from build123d import *

# Parameters (mm, degrees)
BOSS_EXTRU_1_DEPTH = 100
ESQUISSE2_W        = 20
ESQUISSE2_H        = 60
BOSS_EXTRU_2_DEPTH = 40
CONG_1_R           = 10
CONG_2_R           = 10
CONG_3_R           = 10


with BuildPart() as part:
    # Esquisse1 → Boss.-Extru.1 (new body)
    with BuildSketch(Plane.XY):
        with BuildLine():
            Line((90, -10), (90, 10))
            Line((90, 10), (31.994888516, 10))
            ThreePointArc((31.994888516, 10), (10.78168508, 18.786796564), (1.994888516, 40))
            Line((1.994888516, 40), (1.994888516, 88.375065612))
            Line((1.994888516, 88.375065612), (-83.555876775, 88.375065612))
            ThreePointArc((-83.555876775, 88.375065612), (-90.626944587, 85.446133424), (-93.555876775, 78.375065612))
            Line((-93.555876775, 78.375065612), (-93.555876775, 30))
            Line((-93.555876775, 30), (-22.555876775, 30))
            Line((-22.555876775, 30), (-22.555876775, -30))
            Line((-22.555876775, -30), (-93.555876775, -30))
            Line((-93.555876775, -30), (-93.555876775, -78.375065612))
            ThreePointArc((-93.555876775, -78.375065612), (-90.626944587, -85.446133424), (-83.555876775, -88.375065612))
            Line((-83.555876775, -88.375065612), (1.994888516, -88.375065612))
            Line((1.994888516, -88.375065612), (1.994888516, -40))
            ThreePointArc((1.994888516, -40), (10.78168508, -18.786796564), (31.994888516, -10))
            Line((31.994888516, -10), (90, -10))
        make_face()
    extrude(amount=BOSS_EXTRU_1_DEPTH)

    # Esquisse2 → Boss.-Extru.2 (add)
    with BuildSketch(Plane.ZY.offset(22.555876775)):
        with Locations((90, 0)):
            Rectangle(ESQUISSE2_W, ESQUISSE2_H)
    extrude(amount=BOSS_EXTRU_2_DEPTH)

    # Congé1
    cong_1_edges = [part.edges().sort_by_distance(p)[0] for p in [
        (1.994888516, -88.375065612, 50),
    ]]
    fillet(cong_1_edges, radius=CONG_1_R)

    # Congé2
    cong_2_edges = [part.edges().sort_by_distance(p)[0] for p in [
        (1.994888516, 88.375065612, 50),
    ]]
    fillet(cong_2_edges, radius=CONG_2_R)

    # Congé3
    cong_3_edges = [part.edges().sort_by_distance(p)[0] for p in [
        (90, -10, 50),
        (90, 10, 50),
    ]]
    fillet(cong_3_edges, radius=CONG_3_R - 0.0001)  # a hair under: the kernel refuses the full size


solid = part.part
The listing builds one solid part. Answer for the finished solid, in the listing's coordinates (mm). A direction names the side the tool comes from. Give positions to 0.01 mm unless a question says otherwise; leave off trailing zeros. Loops run counter-clockwise (first coordinate to the right, second up) from the corner with the lowest first, then second, coordinate; pieces in that order, holes last. Notation, with made-up numbers: (52, 64) - (108, 64) arc R20 ccw to (108, 69) - close; hole circle Ø5 at (69, 79). An arc over 180 degrees is marked (long way). Answer as a JSON object with one key per item and string values.
1. For a pull along Y with two mould halves and no side action, classify faces 1 (the flat face through (-46, -88.375, 49)), 2 (the flat face through (-93.556, 55, 49)), 3 (the flat face through (-22.556, 0, 39)), 4 (the cylindrical face through (-90.55, 85.52, 49.3)) as pulls with the +Y half, pulls with the -Y half, needs draft (parallel to the pull), parting line crosses it, or undercut.
Determined:
{"face 1": "pulls with the -Y half", "face 2": "needs draft", "face 3": "undercut", "face 4": "pulls with the +Y half"}
2. A cutting plane is placed at C-C (x = -31). Write down the section's boundary in (y, z), then the cut area to 3 significant figures.
Determined:
{"outline": "(-88.38, 0) - (-30, 0) - (-30, 80) - (30, 80) - (30, 0) - (88.38, 0) - (88.38, 100) - (-88.38, 100) - close", "area": "12,900 mm²"}
3. Find the intervals of material crossed by L1, parallel to Y at x = -29, z = 63; L2, parallel to X at y = 60, z = 95.5; L3, parallel to Y at x = 39.5, z = 60, in increasing order. Write a range as [from, to].
Determined:
{"L1": "[-88.38, -30], [30, 88.38]", "L2": "[-93.56, 1.99]", "L3": "[-10, 10]"}
4. For faces 5 (the flat face through (56, -10, 49)), 6 (the flat face through (-59, 30, 49)), 7 (the flat face through (-62.556, 0, 90)), 8 (the flat face through (1.995, 59, 49)), determine the directions among +Z, -Z, +X, -X, +Y, -Y from which every point of the face is accessible in a straight line to the end or side of a thin tool.
Determined:
{"face 5": "+Z, -Z, +X, -Y", "face 6": "-Z, -X", "face 7": "+Z, -Z, -X", "face 8": "+Z, -Z, +X, +Y"}
5. A cutting plane is placed at A-A (x = -80.5). Write down the section's boundary in (y, z), then the cut area to 3 significant figures.
Determined:
{"outline": "(-88.38, 0) - (-30, 0) - (-30, 100) - (-88.38, 100) - close; (30, 0) - (88.38, 0) - (88.38, 100) - (30, 100) - close", "area": "11,700 mm²"}
6. Flat-ended cylindrical pins translate along their axes: pin 1 Ø18 at (y, z) = (4.5, 26.5) entering from -X; pin 2 Ø4 at (x, z) = (40.5, 39) entering from -Y; pin 3 Ø3 at (x, y) = (-58, -27.5) entering from -Z. Find the tip coordinate at first contact, or state that the pin passes through.
Determined:
{"pin 1": "x = -22.56", "pin 2": "y = -10", "pin 3": "z = 80"}
7. A cutting plane is placed at D-D (y = -5.5). Write down the section's boundary in (x, z).
Determined:
{"outline": "(-62.56, 80) - (-22.56, 80) - (-22.56, 0) - (88.35, 0) - (88.35, 100) - (-62.56, 100) - close"}
